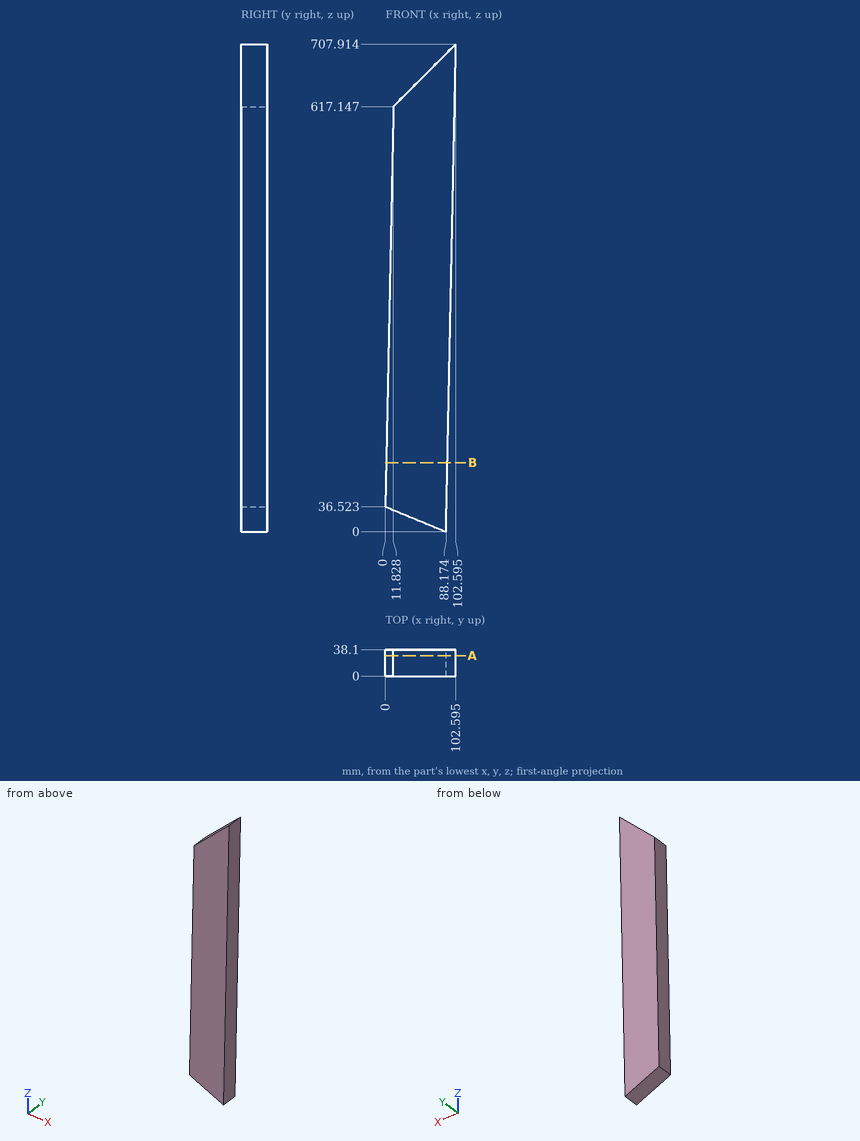
Here's the drawing with two shaded views (mm, measured from the low corner). I have some questions. Coordinates: 2 decimals unless noted, no trailing zeros. Order: outer loops, then holes, each group sorted by start corner. A loop starts at its lowest first (then second) coordinate and runs counter-clockwise, first axis right, second up. Notation, with made-up numbers: (45.5, -21.5) - (94.5, -21.5) arc R17 cw to (94.5, -7.5) - close; hole circle Ø11 at (24, -9). An arc over 180 degrees is marked (long way). Answer in a Markdown table with one row per item. Add a question column.
(1) If we section it at B-B, the plane z = 100.5: Please give me the cut outline in (x, y), then the cut area to 3 significant figures.
(2) Will these pins go through, and if not, where does the flat tip stop? pin 1 (12 mm diameter, centred on x = 12.5, y = 12.5, fed in from +Z); pin 2 (10 mm diameter, centred on y = 25.5, z = 444, fed in from +X); pin 3 (12 mm diameter, centred on y = 28, z = 456, fed in from -X); pin 4 (1.5 mm diameter, centred on x = 88.5, z = 198.5, fed in from -Y).
(3) If we section it at A-A, the plane y = 29.5: Please give me the cut outline in (x, z) (1 decimal).
(4) I need wall thicknesses on L1, parallel to X at y = 23, z = 62; L2, parallel to X at y = 22, z = 486 (1 decimal); L3, parallel to Z at x = 55.5, y = 21 (1 decimal). Which ranges of each line are inside material? Lowest first, please.
Results are:
| question | item | result |
|---|---|---|
| 1 | outline | (1.3, 0) - (90.22, 0) - (90.22, 38.1) - (1.3, 38.1) - close |
| 1 | area | 3,390 mm2 |
| 2 | pin 1 | stops at z = 623.82 |
| 2 | pin 2 | stops at x = 97.32 |
| 2 | pin 3 | stops at x = 8.42 |
| 2 | pin 4 | stops at y = 0 |
| 3 | outline | (0, 36.5) - (88.2, 0) - (102.6, 707.9) - (11.8, 617.1) - close |
| 4 | L1 | x = 0.52 to 89.44 |
| 4 | L2 | x = 9.2 to 98.1 |
| 4 | L3 | z = 13.5 to 660.8 |
